Part model, mm, in its own coordinate system. Face numbers are marked on the shaded views. A direction names the side the tool comes from. Round coordinates to 2 decimals unless told otherwise and drop trailing zeros. Write each loop counter-clockwise with the first axis right and the second up, starting at its lowest first coordinate (ties: lowest second). Pieces come first, ordered by that corner, then holes.
1) Flat gauge pins, fed straight in: pin 1 (10.5 mm diameter, centred on y = 2, z = -12.5, fed in from +X); pin 2 (1.5 mm diameter, centred on y = -0.5, z = -10, fed in from +X); pin 3 (2 mm diameter, centred on y = -0.5, z = -4.5, fed in from +X); pin 4 (8 mm diameter, centred on x = 17.5, y = 4.5, fed in from -Z). Where does each tip first touch, or does it go through?
2) Drill centre lines: L1, parallel to Z at x = 24.5, y = 3; L2, parallel to X at y = 3.5, z = -14.5; L3, parallel to Y at x = -19.85, z = -0.5. Where is each one in solid material? Low to high.
3) Saw through at C-C on y = 1.5. Write the cut outline in (x, z).
4) Which spindle directions (+Z, -Z, +X, -X, +Y, -Y) get a long thin tool onto all of the face, cutting with end or side? Do the marked faces 4 and 5. Say none if no direction does.
5) Saw through at A-A on x = 9. Write the cut outline in (y, z).
6) Saw through at B-B on z = 0.25. Write the cut outline in (x, y).
7) Pull direction Y, two halves, no side cores. Call the marked faces 1, 2 and 3: +Y half, -Y half, draft (parallel to the pull), parting line (faces both ways), or undercut.
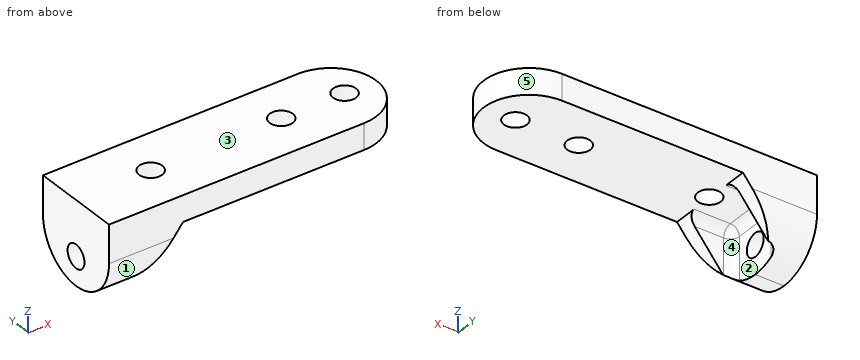
```python
from build123d import *

# Parameters (mm, degrees)
BOSS_EXTRUDE1_DEPTH     = 2.8575
CUT_EXTRUDE1_DEPTH      = 33.135046678
CUT_EXTRUDE1_DEPTH_BACK = 33.135046678
SKETCH3_R               = 2.55
SKETCH4_R               = 2.55
CUT_EXTRUDE2_DEPTH      = 5.715
SKETCH5_W               = 18.318839082
SKETCH5_H               = 20
BOSS_EXTRUDE2_DEPTH     = 6.35
FILLET1_R               = 10
CUT_EXTRUDE3_DEPTH      = 69.857646679
CUT_EXTRUDE3_DEPTH_BACK = 69.857646679
SKETCH6_R               = 2.55
BOSS_EXTRUDE3_DEPTH     = 3.175
CUT_EXTRUDE4_DEPTH      = 69.857646679
CUT_EXTRUDE4_DEPTH_BACK = 69.857646679
FILLET2_R               = 2


with BuildPart() as part:
    # Sketch2 → Boss-Extrude1 (new, symmetric)
    with BuildSketch(Plane.XY):
        with BuildLine():
            Line((-30, 10), (-30, -10))
            Line((-30, -10), (20, -10))
            ThreePointArc((20, -10), (30, 0), (20, 10))
            Line((20, 10), (-30, 10))
        make_face()
    extrude(amount=BOSS_EXTRUDE1_DEPTH, both=True)

    # Sketch3 → Cut-Extrude1 (cut, two sides: drawn at the far end of the back side and taken through both)
    with BuildSketch(Plane.XY.offset(2.8575).offset(-CUT_EXTRUDE1_DEPTH_BACK)):
        with Locations((9, 0)):
            Circle(SKETCH3_R)
        with Locations((23, 0)):
            Circle(SKETCH3_R)
    extrude(amount=CUT_EXTRUDE1_DEPTH + CUT_EXTRUDE1_DEPTH_BACK, mode=Mode.SUBTRACT)

    # Sketch4 → Cut-Extrude2 (cut)
    with BuildSketch(Plane.XY.offset(2.8575)):
        with Locations((-19.85, 0)):
            Circle(SKETCH4_R)
    extrude(amount=-CUT_EXTRUDE2_DEPTH, mode=Mode.SUBTRACT)

    # Sketch5 → Boss-Extrude2 (add)
    with BuildSketch(Plane.ZY.offset(30)):
        with Locations((-6.301919541, 0)):
            Rectangle(SKETCH5_W, SKETCH5_H)
    extrude(amount=BOSS_EXTRUDE2_DEPTH)

    # Fillet1
    fillet1_edges = [part.edges().sort_by_distance(p)[0] for p in [
        (-33.175, -10, -15.461339082),
        (-33.175, 10, -15.461339082),
    ]]
    fillet(fillet1_edges, radius=FILLET1_R - 0.0001)  # a hair under: the kernel refuses the full size

    # Sketch6 → Cut-Extrude3 (cut, two sides: drawn at the far end of the back side and taken through both)
    with BuildSketch(Plane.ZY.offset(36.35).offset(-CUT_EXTRUDE3_DEPTH_BACK)):
        with Locations(Location((-9.1425, 0, 0), (0, 0, 90))):
            Circle(SKETCH6_R)
    extrude(amount=CUT_EXTRUDE3_DEPTH + CUT_EXTRUDE3_DEPTH_BACK, mode=Mode.SUBTRACT)

    # Sketch7 → Boss-Extrude3 (add)
    with BuildSketch(Plane(origin=(0, 10, 0), x_dir=(1, 0, 0), z_dir=(0, 1, 0))):
        Polygon((-30, 2.8575), (-20, 2.8575), (-30, 15.461339082), (-30, 5.461339082), align=None)
    boss_extrude3 = extrude(amount=-BOSS_EXTRUDE3_DEPTH)

    # Mirror1: Boss-Extrude3 across plane
    add(boss_extrude3.mirror(Plane.ZX))

    # Sketch8 → Cut-Extrude4 (cut, two sides: drawn at the far end of the back side and taken through both)
    with BuildSketch(Plane.ZY.offset(36.35).offset(-CUT_EXTRUDE4_DEPTH_BACK)):
        with BuildLine():
            ThreePointArc((-15.461339082, 0), (-12.532406894, 7.071067812), (-5.461339082, 10))
            Line((-5.461339082, 10), (-15.461339082, 10))
            Line((-15.461339082, 10), (-15.461339082, 0))
        make_face()
        with BuildLine():
            Line((-15.461339082, -10), (-5.461339082, -10))
            ThreePointArc((-5.461339082, -10), (-12.532406894, -7.071067812), (-15.461339082, 0))
            Line((-15.461339082, 0), (-15.461339082, -10))
        make_face()
    extrude(amount=CUT_EXTRUDE4_DEPTH + CUT_EXTRUDE4_DEPTH_BACK, mode=Mode.SUBTRACT)

    # Fillet2
    fillet2_edges = [part.edges().sort_by_distance(p)[0] for p in [
        (-30, 0, -2.8575),
        (-30, 6.825, -7.813847506),
        (-25, 6.825, -2.8575),
        (-30, -6.825, -7.813847506),
        (-25, -6.825, -2.8575),
    ]]
    fillet(fillet2_edges, radius=FILLET2_R)


solid = part.part
```
Completed:
1. pin 1: stops at x = -26.01
1. pin 2: passes through
1. pin 3: stops at x = -29.47
1. pin 4: stops at z = -2.86
2. L1: z = -2.86 to 2.86
2. L2: x = -36.35 to -30
2. L3: y = -10 to -2.55, 2.55 to 10
3. outline: (-36.35, -15.35) - (-30, -15.35) - (-30, -11.2) - (-36.35, -11.2) - close; (-36.35, -7.08) - (-30, -7.08) - (-30, -4.86) arc R2 cw to (-28, -2.86) - (-21.91, -2.86) - (-21.91, 2.86) - (-36.35, 2.86) - close; (-17.79, -2.86) - (6.94, -2.86) - (6.94, 2.86) - (-17.79, 2.86) - close; (11.06, -2.86) - (20.94, -2.86) - (20.94, 2.86) - (11.06, 2.86) - close; (25.06, -2.86) - (29.89, -2.86) - (29.89, 2.86) - (25.06, 2.86) - close
4. face 4: -Z, +X
4. face 5: +Z, -Z, +X
5. outline: (-10, -2.86) - (-2.55, -2.86) - (-2.55, 2.86) - (-10, 2.86) - close; (2.55, -2.86) - (10, -2.86) - (10, 2.86) - (2.55, 2.86) - close
6. outline: (-36.35, -10) - (20, -10) arc R10 ccw to (20, 10) - (-36.35, 10) - close; hole circle Ø5.1 at (-19.85, 0); hole circle Ø5.1 at (9, 0); hole circle Ø5.1 at (23, 0)
7. face 1: -Y half
7. face 2: undercut
7. face 3: draft
